from build123d import *

# Parameters (mm, degrees)
SKETCH1_W           = 6
SKETCH1_H           = 6
BOSS_EXTRUDE1_DEPTH = 8.31
SKETCH2_R           = 2.125
CUT_EXTRUDE1_DEPTH  = 10
SKETCH3_R           = 3.75
BOSS_EXTRUDE2_DEPTH = 50


with BuildPart() as part:
    # Sketch1 → Boss-Extrude1 (new body)
    with BuildSketch(Plane(origin=(0, 0, 0), x_dir=(1, 0, 0), z_dir=(0, 1, 0))):
        with Locations((3, 3)):
            Rectangle(SKETCH1_W, SKETCH1_H)
    extrude(amount=BOSS_EXTRUDE1_DEPTH)

    # Sketch2 → Cut-Extrude1 (cut)
    with BuildSketch(Plane(origin=(6, 0, 0), x_dir=(0, 0, -1), z_dir=(1, 0, 0))):
        with Locations((3, 3.31)):
            Circle(SKETCH2_R)
    extrude(amount=-CUT_EXTRUDE1_DEPTH, mode=Mode.SUBTRACT)

    # Sketch3 → Boss-Extrude2 (add)
    with BuildSketch(Plane(origin=(0, 8.31, 0), x_dir=(1, 0, 0), z_dir=(0, 1, 0))):
        with Locations((3, 3)):
            Circle(SKETCH3_R)
    extrude(amount=BOSS_EXTRUDE2_DEPTH)


solid = part.part
Read the model definition and answer for the solid it produces. Units are mm, in the model's axes. A direction names the side the tool comes from. Give positions to 0.01 mm unless a question says otherwise; leave off trailing zeros. Loops run counter-clockwise (first coordinate to the right, second up) from the corner with the lowest first, then second, coordinate; pieces in that order, holes last. Notation, with made-up numbers: (7, 15.5) -> (15, 15.5) arc R26 cw to (15, 53.5) -> close; hole circle Ø7 at (73, 42.5). An arc over 180 degrees is marked (long way). Use a Markdown table: item, result.
Q1. A tool of negligible diameter and unlimited length cuts with its end or side. For faces 4 (the face through (3, 4, 0)), 5 (the face through (2.512, 32.96, -6.718)), 6 (the face through (6, 6, -3)), from which of +Z, -Z, +X, -X, +Y, -Y can it reach the whole face along a straight path? Write none if from no direction.
Solved:
| item | result |
|---|---|
| face 4 | +Z, +X, -X, -Y |
| face 5 | +Y |
| face 6 | +Z, -Z, +X, -Y |
Q2. Each of these flat-tipped pins is pushed along its axis until it touches: pin 1 (0.8 mm diameter, centred on x = 3, z = 0.5, fed in from -Y); pin 2 (1.8 mm diameter, centred on x = 1.5, y = 6, fed in from -Z); pin 3 (1.8 mm diameter, centred on x = 3.5, y = 3, fed in from +Z). Where does it stop, or does it pass through?
Solved:
| item | result |
|---|---|
| pin 1 | stops at y = 8.31 |
| pin 2 | stops at z = -6 |
| pin 3 | stops at z = 0 |
Q3. Determine the mould class of faces 1 (the face through (3.04, 2.02, -1.31)), 2 (the face through (3, 4, -6)), 3 (the face through (3, 58.31, -3)) for opening direction Y: pulls with the +Y half, pulls with the -Y half, needs draft (parallel to the pull), parting line crosses it, or undercut.
Solved:
| item | result |
|---|---|
| face 1 | undercut |
| face 2 | needs draft |
| face 3 | pulls with the +Y half |
Q4. Section B-B, the plane x = 3 is taken. Determine the outline of the cut face in (y, z) (3 decimals).
Solved:
| item | result |
|---|---|
| outline | (0, -6) -> (8.31, -6) -> (8.31, -6.75) -> (58.31, -6.75) -> (58.31, 0.75) -> (8.31, 0.75) -> (8.31, 0) -> (0, 0) -> close; hole circle Ø4.25 at (3.31, -3) |
Q5. Section C-C, the plane z = -3 is taken. Determine the outline of the cut face in (x, y) (3 decimals).
Solved:
| item | result |
|---|---|
| outline | (-0.75, 8.31) -> (0, 8.31) -> (0, 5.435) -> (6, 5.435) -> (6, 8.31) -> (6.75, 8.31) -> (6.75, 58.31) -> (-0.75, 58.31) -> close; (0, 0) -> (6, 0) -> (6, 1.185) -> (0, 1.185) -> close |
Q6. Find the intervals of material crossed by line 1 along Y through (x, z) = (3.15, -3) (3 decimals); line 2 along X through (y, z) = (14, -2.75); line 3 along Y through (x, z) = (4.5, -3.75), in increasing order.
Solved:
| item | result |
|---|---|
| line 1 | y = 0 to 1.185, 5.435 to 58.31 |
| line 2 | x = -0.74 to 6.74 |
| line 3 | y = 0 to 1.32, 5.3 to 58.31 |
Q7. Section D-D, the plane y = 48 is taken. Determine the outline of the cut face in (x, z), then the cut area to 3 significant figures.
Solved:
| item | result |
|---|---|
| outline | circle Ø7.5 at (3, -3) |
| area | 44.2 mm^2 |
Q8. Section A-A, the plane y = 3.31 is taken. Determine the outline of the cut face in (x, z) (3 decimals), then the cut area to 3 significant figures.
Solved:
| item | result |
|---|---|
| outline | (0, -6) -> (6, -6) -> (6, -5.125) -> (0, -5.125) -> close; (0, -0.875) -> (6, -0.875) -> (6, 0) -> (0, 0) -> close |
| area | 10.5 mm^2 |
